```python
from build123d import *

# Parameters (mm, degrees)
F0_W     = 175.017152
F0_H     = 175.017152
F0_R     = 1.7272
F0_R_2   = 12.7
F1_DEPTH = 5.08


with BuildPart() as f1:
    # F0 (on Top) → F1 (new body)
    with BuildSketch(Plane.XY):
        Rectangle(F0_W, F0_H)
        with Locations((-81.158576, -82.746076)):
            Circle(F0_R, mode=Mode.SUBTRACT)
        with Locations((-81.158576, -63.696076)):
            Circle(F0_R, mode=Mode.SUBTRACT)
        with Locations((-12.909118, -12.909118)):
            Circle(F0_R, mode=Mode.SUBTRACT)
        with Locations((81.158576, -82.746076)):
            Circle(F0_R, mode=Mode.SUBTRACT)
        with Locations((81.158576, -63.696076)):
            Circle(F0_R, mode=Mode.SUBTRACT)
        with Locations((12.909118, -12.909118)):
            Circle(F0_R, mode=Mode.SUBTRACT)
        with Locations((-12.909118, 12.909118)):
            Circle(F0_R, mode=Mode.SUBTRACT)
        with Locations((-24.892, 38.548238)):
            Circle(F0_R, mode=Mode.SUBTRACT)
        with Locations((-81.158576, 63.696076)):
            Circle(F0_R, mode=Mode.SUBTRACT)
        with Locations((-81.158576, 82.746076)):
            Circle(F0_R, mode=Mode.SUBTRACT)
        with Locations((-24.892, 48.327238)):
            Circle(F0_R, mode=Mode.SUBTRACT)
        Circle(F0_R_2, mode=Mode.SUBTRACT)
        with Locations((12.909118, 12.909118)):
            Circle(F0_R, mode=Mode.SUBTRACT)
        with BuildLine():
            Line((-20.32, 44.453738), (-20.32, 53.216738))
            Line((-20.32, 53.216738), (20.32, 53.216738))
            Line((20.32, 53.216738), (20.32, 44.453738))
            Line((20.32, 44.453738), (23.749, 44.453738))
            ThreePointArc((23.749, 44.453738), (24.765, 43.437738), (23.749, 42.421738))
            Line((23.749, 42.421738), (20.32, 42.421738))
            Line((20.32, 42.421738), (20.32, 33.658738))
            Line((20.32, 33.658738), (-20.32, 33.658738))
            Line((-20.32, 33.658738), (-20.32, 42.421738))
            Line((-20.32, 42.421738), (-23.749, 42.421738))
            ThreePointArc((-23.749, 42.421738), (-24.765, 43.437738), (-23.749, 44.453738))
            Line((-23.749, 44.453738), (-20.32, 44.453738))
        make_face(mode=Mode.SUBTRACT)
        with Locations((24.892, 38.548238)):
            Circle(F0_R, mode=Mode.SUBTRACT)
        with Locations((24.892, 48.327238)):
            Circle(F0_R, mode=Mode.SUBTRACT)
        with Locations((81.158576, 63.696076)):
            Circle(F0_R, mode=Mode.SUBTRACT)
        with Locations((81.158576, 82.746076)):
            Circle(F0_R, mode=Mode.SUBTRACT)
    extrude(amount=F1_DEPTH)


solid = f1.part
```
Can you work these out from the model? Positions are in its coordinate system, mm. A direction names the side the tool comes from. Coordinates: 2 decimals unless noted, no trailing zeros. Loops run counter-clockwise (first coordinate to the right, second up) from the corner with the lowest first, then second, coordinate; pieces in that order, holes last. Notation, with made-up numbers: (-35.5, -12.5) -> (-31.5, -12.5) arc R8 cw to (-31.5, -7.5) -> close; hole circle Ø9 at (16.5, 74). An arc over 180 degrees is marked (long way). Answer as a JSON object with one key per item and string values.
1) Imagine slicing it at A-A (y = 0). Please give me the cut outline in (x, z), then the cut area to 3 significant figures.
Results:
{"outline": "(-87.51, 0) -> (-12.7, 0) -> (-12.7, 5.08) -> (-87.51, 5.08) -> close; (12.7, 0) -> (87.51, 0) -> (87.51, 5.08) -> (12.7, 5.08) -> close", "area": "760 mm^2"}
2) For P1, Ø3, axis at x = -24.89, y = 48.33, coming from the +Z side, with a flat end and sliding along its axis, tell me the tip position at first contact or that it passes through.
Results:
{"P1": "passes through"}
3) Thinking about a two-plate mould opening in Y: for faces 1 (the face through (20.32, 38, 3)), 2 (the face through (-1, 87.509, 3)), 3 (the face through (20.32, 49, 3)), 4 (the face through (-87.509, -1, 3)), which applies, pulls with the +Y half, pulls with the -Y half, needs draft (parallel to the pull), parting line crosses it, or undercut?
Results:
{"face 1": "undercut", "face 2": "pulls with the +Y half", "face 3": "undercut", "face 4": "needs draft"}
4) For faces 5 (the face through (-20.32, 49, 3)), 6 (the face through (-1, -18, 5.08)), which set-ups out of +Z, -Z, +X, -X, +Y, -Y let a thin tool reach every point of the face, with its end or its side?
Results:
{"face 5": "+Z, -Z", "face 6": "+Z, +X, -X, +Y, -Y"}
5) Imagine slicing it at B-B (x = 0). Please give me the cut outline in (y, z).
Results:
{"outline": "(-87.51, 0) -> (-12.7, 0) -> (-12.7, 5.08) -> (-87.51, 5.08) -> close; (12.7, 0) -> (33.66, 0) -> (33.66, 5.08) -> (12.7, 5.08) -> close; (53.22, 0) -> (87.51, 0) -> (87.51, 5.08) -> (53.22, 5.08) -> close"}
6) Imagine slicing it at C-C (z = 4.25). Count the separate pieces of the cut face and the enclosed holes in it, then the cut area to 3 significant figures.
Results:
{"separate pieces": "1", "enclosed holes": "18", "area": "29,200 mm^2"}
7) If I drill on line 1 (X direction, y = -63.5, z = 2.7); line 2 (X direction, y = 34.5, z = 2.8); line 3 (X direction, y = 13, z = 0.6), over which ranges is the centre line in solid material (lowest first)?
Results:
{"line 1": "x = -87.51 to -82.87, -79.44 to 79.44, 82.87 to 87.51", "line 2": "x = -87.51 to -20.32, 20.32 to 87.51", "line 3": "x = -87.51 to -14.63, -11.18 to 11.18, 14.63 to 87.51"}
